Autodesk Inventor part; units mm, degrees
ref_plane "YZ Plane" through (0, 0, 0) normal (1, 0, 0) x (0, 1, 0)
ref_plane "XZ Plane" through (0, 0, 0) normal (0, 1, 0) x (-1, 0, 0)
ref_plane "XY Plane" through (0, 0, 0) normal (0, 0, 1) x (1, 0, 0)
sketch "Sketch1" plane through (0, 0, 0) normal (1, 0, 0) x (0, 1, 0)
  line L0 (0, 0) -> (65, 0)
  line L1 (65, 0) -> (65, -40)
  line L2 (65, -40) -> (0, -40)
  line L3 (0, -40) -> (0, 0)
  dimension "d0" = 40
  dimension "d1" = 65
extrude "Extrusion1" add sketch "Sketch1" along normal blind 3
sketch "Sketch2" plane through (0, 0, 0) normal (-1, 0, 0) x (0, 0, 1)
  line L0 (0, 0) -> (-40, 0)
  line L1 (-40, 0) -> (-40, 65)
  line L2 (0, 0) -> (-40, 0)
  line L3 (-40, 0) -> (-40, 5)
  line L4 (-40, 5) -> (0, 5)
  line L5 (0, 5) -> (0, 0)
  dimension "d4" = 5
extrude "Extrusion2" add sketch "Sketch2" along normal blind 20
chamfer "Chamfer1" distance 10 angle 45 1 edges at (0, 5, -20)
sketch "Sketch3" plane through (3, 0, 0) normal (1, 0, 0) x (0, 0, -1)
  circle A0 centre (20, 55) radius 5
  circle A1 centre (20, 40) radius 5
  circle A2 centre (20, 25) radius 5
  line L0 (40, 65) -> (0, 65)
  point P0 (0, 0)
  dimension "d10" = 10
  dimension "d11" = 10
  dimension "d12" = 5
  dimension "d13" = 15
  dimension "d14" = 20
extrude "Extrusion3" cut sketch "Sketch3" against normal up to surface (3 mm away)
fillet "Fillet1" radius 20 2 edges at (1.5, 65, 0) (1.5, 65, -40)
properties part number "pot_stand"
Here's how the part is built. I have some questions about the finished solid (model axes, mm). A direction names the side the tool comes from. Coordinates: 2 decimals unless noted, no trailing zeros. Order: outer loops, then holes, each group sorted by start corner. A loop starts at its lowest first (then second) coordinate and runs counter-clockwise, first axis right, second up.
Item 1: I need wall thicknesses on probe 1 along Y at (x, z) = (1, -20); probe 2 along X at (y, z) = (16, -33); probe 3 along Y at (x, z) = (-12.5, -38). Which ranges of each line are inside material? Lowest first, please.
Response values:
probe 1: y = 0 to 20, 30 to 35, 45 to 50, 60 to 65
probe 2: x = 0 to 3
probe 3: y = 0 to 5
Item 2: Thinking about a two-plate mould opening in Z: for faces 1 (the face through (1.521, 59.297, -6.014)), 2 (the face through (1.521, 58.986, -34.297)), 3 (the face through (1.521, 44.957, -19.349)), which applies, pulls with the +Z half, pulls with the -Z half, needs draft (parallel to the pull), parting line crosses it, or undercut?
Response values:
face 1: pulls with the +Z half
face 2: pulls with the -Z half
face 3: undercut
Item 3: If we section it at A-A, the plane x = 0.75: Give the number of separate pieces and of enclosed holes in the cut face, then the cut area to 3 significant figures.
Response values:
separate pieces: 1
enclosed holes: 3
area: 2,190 mm2
Item 4: If we section it at B-B, the plane y = 40: List the corners of the cut face in (x, z) for me.
Response values:
outline: (0, -40) - (3, -40) - (3, -25) - (0, -25) - close; (0, -15) - (3, -15) - (3, 0) - (0, 0) - close
Item 5: Which directions (+Z, -Z, +X, -X, +Y, -Y) give clear straight access to the entire face, cutting with the end or side of a thin tool? Please do faces 4 (the face through (1.521, 59.957, -19.349)), 5 (the face through (0, 34, -20)).
Response values:
face 4: +X, -X
face 5: +Z, -Z, -X, +Y
Item 6: If we section it at C-C, the plane z = -18: List the corners of the cut face in (x, y) for me.
Response values:
outline: (-20, 0) - (3, 0) - (3, 20.42) - (0, 20.42) - (0, 15) - (-10, 5) - (-20, 5) - close; (0, 29.58) - (3, 29.58) - (3, 35.42) - (0, 35.42) - close; (0, 44.58) - (3, 44.58) - (3, 50.42) - (0, 50.42) - close; (0, 59.58) - (3, 59.58) - (3, 64.9) - (0, 64.9) - close
Item 7: If we section it at D-D, the plane y = 28: List the corners of the cut face in (x, z) for me.
Response values:
outline: (0, -40) - (3, -40) - (3, -24) - (0, -24) - close; (0, -16) - (3, -16) - (3, 0) - (0, 0) - close
Item 8: I'm going to push flat-ended pins straight in: pin 1 Ø11.5 at (y, z) = (40, -20) entering from -X; pin 2 Ø8 at (x, z) = (-14.5, -25) entering from +Y; pin 3 Ø4 at (x, z) = (-11, -14) entering from +Y; pin 4 Ø3 at (x, z) = (-1.5, -12.5) entering from -Y. Where does each tip first touch, or does it pass through?
Response values:
pin 1: stops at x = 0
pin 2: stops at y = 5
pin 3: stops at y = 6
pin 4: stops at y = 0
